Read the model definition and answer for the solid it produces. Units are mm, in the model's axes. Face numbers are marked on the shaded views. A direction names the side the tool comes from. Give positions to 0.01 mm unless a question says otherwise; leave off trailing zeros. Loops run counter-clockwise (first coordinate to the right, second up) from the corner with the lowest first, then second, coordinate; pieces in that order, holes last.
(1) Straight lines are drawn through the part: probe 1 along Z at (x, y) = (1.5, 5.75); probe 2 along Z at (x, y) = (-6.5, -4.5); probe 3 along Y at (x, z) = (4, 28.5). For each, find the intervals that lie inside material, in ascending order.
(2) Each of these flat-tipped pins is pushed along its axis until it touches: P1, Ø3, axis at x = 5.5, y = 6, coming from the +Z side; P2, Ø1.5, axis at y = -1, z = 23, coming from the -X side; P3, Ø10, axis at x = 6, z = 20, coming from the +Y side. Where does it stop, or does it pass through?
(3) Find section A-A, the plane x = 0. Write down the section's boundary in (y, z), then the cut area to 3 significant figures.
(4) Which of the six approach directions +Z, -Z, +X, -X, +Y, -Y give full straight-line access (tool end or side, diameter ignored) to the marked faces 1 and 2?
(5) Find section C-C, the plane z = 15. Write down the section's boundary in (x, y), then the cut area to 3 significant figures.
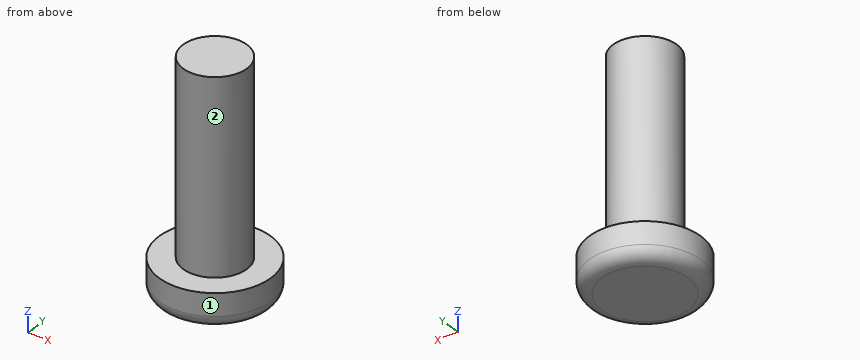
```python
from build123d import *

# Parameters (mm, degrees)
SKETCH_1_R      = 5
EXTRUDE_1_DEPTH = 30
SKETCH_2_R      = 8.75
EXTRUDE_2_DEPTH = 5.5
FILLET_2_R      = 2


with BuildPart() as part:
    # 草图1 → 凸台-拉伸1 (new body)
    with BuildSketch(Plane.XY):
        Circle(SKETCH_1_R)
    extrude(amount=EXTRUDE_1_DEPTH)

    # Sketch 2 → 凸台-拉伸2 (add)
    with BuildSketch(Plane(origin=(0, 0, 0), x_dir=(-1, 0, 0), z_dir=(0, 0, -1))):
        Circle(SKETCH_2_R)
    extrude(amount=EXTRUDE_2_DEPTH)

    # 圆角2
    fillet_2_edges = [part.edges().sort_by_distance(p)[0] for p in [
        (8.75, 0, -5.5),
    ]]
    fillet(fillet_2_edges, radius=FILLET_2_R)


solid = part.part
```
Entries:
1. probe 1: z = -5.5 to 0
1. probe 2: z = -5.13 to 0
1. probe 3: y = -3 to 3
2. P1: stops at z = 0
2. P2: stops at x = -4.99
2. P3: stops at y = 4.9
3. outline: (-8.75, -3.5) arc R2 ccw to (-6.75, -5.5) - (6.75, -5.5) arc R2 ccw to (8.75, -3.5) - (8.75, 0) - (5, 0) - (5, 30) - (-5, 30) - (-5, 0) - (-8.75, 0) - close
3. area: 395 mm2
4. face 1: +Z, -Z
4. face 2: +Z
5. outline: circle Ø10 at (0, 0)
5. area: 78.5 mm2
